Geometry check sheet. Reference: the model listing, model coordinates, mm. Give positions to 0.01 mm unless a question says otherwise; leave off trailing zeros. Write each loop counter-clockwise with the first axis right and the second up, starting at its lowest first coordinate (ties: lowest second). Pieces come first, ordered by that corner, then holes. Notation, with made-up numbers: (-27.5, 46.25) - (-14.5, 46.25) arc R35 ccw to (-14.5, 81.25) - close; hole circle Ø10 at (-25.75, -8.75). An arc over 180 degrees is marked (long way). One line per question, with ' | ' between items. Start each with the question number.
Q1. Thickness scan on L1, parallel to Y at x = 3.25, z = -53; L2, parallel to X at y = 1, z = -119.5; L3, parallel to X at y = 3.9, z = -181.5. Record the ranges inside material, lowest first. Write a range as [from, to].
Q2. Section check A-A on z = -109. Record the boundary of the cut face in (x, y).
Q3. Gauge pin test, flat end, axial feed: P1, Ø4.5, axis at x = 0, z = -120, coming from the +Y side. Record the tip position at first contact, or that the pin passes through.
Autodesk Inventor part; units mm, degrees
ref_plane "rail_to_adjusting_block_XY" through (0, 0, -220) normal (0, 1, 0) x (1, 0, 0)
ref_plane "rail_to_adjusting_block_YZ" through (0, 0, -220) normal (1, 0, 0) x (0, 0, -1)
ref_plane "rail_to_adjusting_block_ZX" through (0, 0, -220) normal (0, 0, -1) x (0, 1, 0)
sketch "Sketch_12" plane through (0, 0, 0) normal (0, 0, 1) x (1, 0, 0)
  line L0 (-4.5, 5.3) -> (-4.5, 5.0434)
  line L1 (-4.5, 5.0434) -> (-4.2216, 4.8827)
  arc A0 (-3.7548, 4.35) -> (-4.2216, 4.8827) centre (-4.7715, 3.93) ccw
  line L2 (-3.7548, 4.35) -> (-3.1, 4.35)
  line L3 (-3.1, 4.35) -> (-3.1, 3.65)
  line L4 (-3.1, 3.65) -> (-3.7548, 3.65)
  arc A1 (-4.2216, 3.1173) -> (-3.7548, 3.65) centre (-4.7715, 4.07) ccw
  line L5 (-4.2216, 3.1173) -> (-4.5, 2.9566)
  line L6 (-4.5, 2.9566) -> (-4.5, 0.3)
  line L7 (-4.5, 0.3) -> (-4.2, 0)
  line L8 (-4.2, 0) -> (4.2, 0)
  line L9 (4.2, 0) -> (4.5, 0.3)
  line L10 (4.5, 0.3) -> (4.5, 2.9566)
  line L11 (4.5, 2.9566) -> (4.2216, 3.1173)
  arc A2 (3.7548, 3.65) -> (4.2216, 3.1173) centre (4.7715, 4.07) ccw
  line L12 (3.7548, 3.65) -> (3.1, 3.65)
  line L13 (3.1, 3.65) -> (3.1, 4.35)
  line L14 (3.1, 4.35) -> (3.7548, 4.35)
  arc A3 (4.2216, 4.8827) -> (3.7548, 4.35) centre (4.7715, 3.93) ccw
  line L15 (4.2216, 4.8827) -> (4.5, 5.0434)
  line L16 (4.5, 5.0434) -> (4.5, 5.3)
  line L17 (4.5, 5.3) -> (4.3, 5.5)
  line L18 (4.3, 5.5) -> (-4.3, 5.5)
  line L19 (-4.3, 5.5) -> (-4.5, 5.3)
extrude "Extrusion1" add sketch "Sketch_12" along normal mid plane 455
sketch "Sketch2" plane through (-4.3, 5.5, 227.5) normal (0, 1, 0) x (1, 0, 0)
  point P0 (4.3, 447.5)
hole "Hole1" at (0, 5.5, -220) direction (0, -1, 0) diameter 3.5 depth 5.5 counterbore diameter 6 counterbore depth 3.5
pattern_linear "Rectangular Pattern1" count 23 spacing 20 along (0, 0, 1) of "Hole1"
ref_plane "rail_to_adjusting_block_XY" through (0, 0, -220) normal (0, 1, 0) x (1, 0, 0)
ref_plane "rail_to_adjusting_block_YZ" through (0, 0, -220) normal (1, 0, 0) x (0, 0, -1)
ref_plane "rail_to_adjusting_block_ZX" through (0, 0, -220) normal (0, 0, -1) x (0, 1, 0)
ref_plane "to_block_XY" through (0, 5.5, 113.75) normal (0, 0, 1) x (1, 0, 0)
ref_plane "to_block_YZ" through (0, 5.5, 113.75) normal (1, 0, 0) x (0, 1, 0)
ref_plane "to_block_ZX" through (0, 5.5, 113.75) normal (0, 1, 0) x (0, 0, 1)
ref_plane "to_block_2_XY" through (0, 5.5, -113.75) normal (0, 0, 1) x (1, 0, 0)
ref_plane "to_block_2_YZ" through (0, 5.5, -113.75) normal (1, 0, 0) x (0, 1, 0)
ref_plane "to_block_2_ZX" through (0, 5.5, -113.75) normal (0, 1, 0) x (0, 0, 1)
ref_plane "to_kue_XY" through (0, 0, 0) normal (0, 1, 0) x (1, 0, 0)
ref_plane "to_kue_YZ" through (0, 0, 0) normal (1, 0, 0) x (0, 0, -1)
ref_plane "to_kue_ZX" through (0, 0, 0) normal (0, 0, -1) x (0, 1, 0)
properties part number "SSE2B-MX10-455_r"
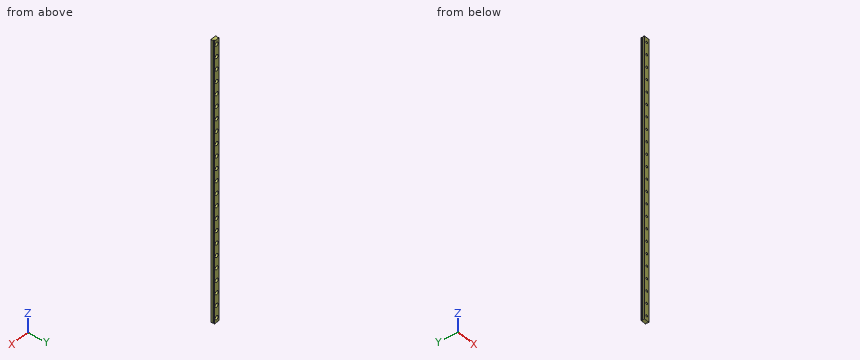
Working result:
1) L1: y = [0, 3.65], [4.35, 5.5] | L2: x = [-4.5, -1.68], [1.68, 4.5] | L3: x = [-3.1, -2.6], [2.6, 3.1]
2) outline: (-4.5, 0.3) - (-4.2, 0) - (4.2, 0) - (4.5, 0.3) - (4.5, 2.96) - (4.22, 3.12) arc R1.1 cw to (3.75, 3.65) - (3.1, 3.65) - (3.1, 4.35) - (3.75, 4.35) arc R1.1 cw to (4.22, 4.88) - (4.5, 5.04) - (4.5, 5.3) - (4.3, 5.5) - (-4.3, 5.5) - (-4.5, 5.3) - (-4.5, 5.04) - (-4.22, 4.88) arc R1.1 cw to (-3.75, 4.35) - (-3.1, 4.35) - (-3.1, 3.65) - (-3.75, 3.65) arc R1.1 cw to (-4.22, 3.12) - (-4.5, 2.96) - close
3) P1: stops at y = 2
